Design review of the part built by this model. Coordinates are the model's own, in mm. A direction names the side the tool comes from. Give positions to 0.01 mm unless a question says otherwise; leave off trailing zeros. Order: outer loops, then holes, each group sorted by start corner. A loop starts at its lowest first (then second) coordinate and runs counter-clockwise, first axis right, second up. Notation, with made-up numbers: (-1.75, 60) -> (46.25, 60) arc R18 ccw to (46.25, 71) -> close; hole circle Ø3 at (-33.75, 12). An arc over 180 degrees is marked (long way). One line per item, written item: value. Start each with the question number.
1) The part is to be moulded in two halves that separate along X. For faces 1 (the face through (0, 3.3, 5)), 2 (the face through (-1, 3, 7)), 3 (the face through (2.082, 3.503, 0.098)), say which applies: released by +X, released by -X, zero draft, split by the parting line, or undercut.
2) For pin 1 (1 mm diameter, centred on y = -1.5, z = 5, fed in from +X); pin 2 (1 mm diameter, centred on x = 2.5, z = -0.5, fed in from -Y); pin 3 (1 mm diameter, centred on y = 3, z = 0.5, fed in from -X); pin 4 (1.5 mm diameter, centred on x = 0, z = -1, fed in from -Y), all flat-tipped, find the tip position at first contact; note any pin that passes through.
3) Consider section B-B (x = 0). State the section outline as (y, z) points (3 decimals), plus the area to 3 significant figures.
4) Consider section A-A (y = 0). State the section outline as (x, z) points (3 decimals), plus the area to 3 significant figures.
5) Wall thickness on line 1 along Z through (x, y) = (3.75, 0); line 2 along Y through (x, z) = (-1.75, 5.75); line 3 along Y through (x, z) = (1.5, -6): over which ranges is each line inside the solid? List them lowest first. Write a range as from..to.
6) Tool access review of faces 4 (the face through (3.256, 2.134, -0.07)), 5 (the face through (1.25, 3, 0)), 6 (the face through (-3.256, 2.134, -0.07)): name each direction out of +Z, -Z, +X, -X, +Y, -Y from which nothing blocks a thin tool from reaching the whole face with its end or side.
from build123d import *

# Parameters (mm, degrees)
SKETCH1_R               = 4.075
SKETCH1_R_2             = 2.875
BOSS_EXTRUDE1_DEPTH     = 7
CUT_EXTRUDE2_DEPTH      = 5
CUT_EXTRUDE2_DEPTH_BACK = 5
CUT_EXTRUDE3_DEPTH      = 10.067041965
CUT_EXTRUDE3_DEPTH_BACK = 10.067041965
FILLET2_R               = 0.6
CUT_EXTRUDE4_DEPTH      = 10.067041965
CUT_EXTRUDE4_DEPTH_BACK = 10.067041965
SKETCH6_W               = 2.5
SKETCH6_H               = 10


with BuildPart() as part:
    # Sketch1 → Boss-Extrude1 (new, symmetric)
    with BuildSketch(Plane.XY):
        Circle(SKETCH1_R)
        Circle(SKETCH1_R_2, mode=Mode.SUBTRACT)
    extrude(amount=BOSS_EXTRUDE1_DEPTH, both=True)

    # Sketch4 → Cut-Extrude2 (cut, two sides: drawn at the far end of the back side and taken through both)
    with BuildSketch(Plane(origin=(0, 0, 0), x_dir=(-1, 0, 0), z_dir=(0, 0, -1)).offset(-CUT_EXTRUDE2_DEPTH_BACK)):
        with BuildLine():
            Line((-3.52905352, 2.0375), (0, 0))
            Line((0, 0), (3.52905352, 2.0375))
            ThreePointArc((3.52905352, 2.0375), (0, -4.075), (-3.52905352, 2.0375))
        make_face()
    extrude(amount=CUT_EXTRUDE2_DEPTH + CUT_EXTRUDE2_DEPTH_BACK, mode=Mode.SUBTRACT)

    # Sketch5 → Cut-Extrude3 (cut, two sides: drawn at the far end of the back side and taken through both)
    with BuildSketch(Plane(origin=(0, 0, 0), x_dir=(-1, 0, 0), z_dir=(0, 0, -1)).offset(-CUT_EXTRUDE3_DEPTH_BACK)):
        with BuildLine():
            Line((-2.619359509, -3.121631106), (0, 0))
            Line((0, 0), (2.619359509, -3.121631106))
            ThreePointArc((2.619359509, -3.121631106), (0, -4.075), (-2.619359509, -3.121631106))
        make_face()
    extrude(amount=CUT_EXTRUDE3_DEPTH + CUT_EXTRUDE3_DEPTH_BACK, mode=Mode.SUBTRACT)

    # Fillet2
    fillet2_edges = [part.edges().sort_by_distance(p)[0] for p in [
        (-3.52905352, 2.0375, 0),
        (-2.489823036, 1.4375, 0),
        (3.52905352, 2.0375, 0),
        (2.489823036, 1.4375, 0),
        (-2.619359509, -3.121631106, 6),
        (-1.848014378, -2.202377774, 6),
        (2.619359509, -3.121631106, 6),
        (1.848014378, -2.202377774, 6),
        (-2.619359509, -3.121631106, -6),
        (-1.848014378, -2.202377774, -6),
        (1.848014378, -2.202377774, -6),
        (2.619359509, -3.121631106, -6),
    ]]
    fillet(fillet2_edges, radius=FILLET2_R - 0.0001)  # a hair under: the kernel refuses the full size

    # Sketch6 → Cut-Extrude4 (cut, two sides: drawn at the far end of the back side and taken through both)
    with BuildSketch(Plane(origin=(0, 0, 0), x_dir=(1, 0, 0), z_dir=(0, 1, 0)).offset(-CUT_EXTRUDE4_DEPTH_BACK)):
        Rectangle(SKETCH6_W, SKETCH6_H)
    extrude(amount=CUT_EXTRUDE4_DEPTH + CUT_EXTRUDE4_DEPTH_BACK, mode=Mode.SUBTRACT)


solid = part.part
Checked values:
1. face 1: undercut
1. face 2: zero draft
1. face 3: split by the parting line
2. pin 1: stops at x = 3.95
2. pin 2: stops at y = 1.63
2. pin 3: stops at x = -3.2
2. pin 4: passes through
3. outline: (2.875, -7) -> (4.075, -7) -> (4.075, -5) -> (2.875, -5) -> close; (2.875, 5) -> (4.075, 5) -> (4.075, 7) -> (2.875, 7) -> close
3. area: 4.80 mm^2
4. outline: (-4.075, -7) -> (-2.875, -7) -> (-2.875, -5) -> (-4.075, -5) -> close; (-4.075, 5) -> (-2.875, 5) -> (-2.875, 7) -> (-4.075, 7) -> close; (2.875, -7) -> (4.075, -7) -> (4.075, -5) -> (2.875, -5) -> close; (2.875, 5) -> (4.075, 5) -> (4.075, 7) -> (2.875, 7) -> close
4. area: 9.60 mm^2
5. line 1: z = -7..-5, 5..7
5. line 2: y = 2.28..3.68
5. line 3: y = 2.45..3.79
6. face 4: +X
6. face 5: +Y, -Y
6. face 6: -X
